from build123d import *

# Parameters (mm, degrees)
ESQUISSE3_R          = 17.5
EXTRUSION1_DEPTH     = 10
EXTRUSION3_START     = -35
EXTRUSION3_OUTLINE_R = 10
EXTRUSION3_DEPTH     = 7
ESQUISSE7_W          = 50
ESQUISSE7_H          = 50
EXTRUSION4_DEPTH     = 7
CONG_1_R             = 10


# Read off the part's stored shape, not the designer's step: Extrusion3
with BuildPart() as part:
    # Esquisse1 → Révol.-Mince1 (revolve)
    with BuildSketch(Plane.XY):
        with BuildLine():
            ThreePointArc((0, -30), (30, 0), (0, 30))
            Line((0, 30), (0, 31))
            ThreePointArc((0, 31), (31, 0), (0, -31))
            Line((0, -31), (0, -30))
        make_face()
    revolve(axis=Axis((0, 52.542035398, 0), (0, -1, 0)))

    # Esquisse3 → Extrusion1 (add)
    with BuildSketch(Plane.XY.offset(20)):
        with Locations(Location((0, 0, 0), (0, 0, 180))):
            Circle(ESQUISSE3_R)
    extrude(amount=EXTRUSION1_DEPTH)

    # Extrusion3 outline → Extrusion3 (add)
    with BuildSketch(Plane(origin=(0, 0, 0), x_dir=(1, 0, 0), z_dir=(0, 1, 0)).offset(EXTRUSION3_START)):
        Circle(EXTRUSION3_OUTLINE_R)
    extrude(amount=EXTRUSION3_DEPTH)

    # Esquisse7 → Extrusion4 (add)
    with BuildSketch(Plane.XZ.offset(35)):
        Rectangle(ESQUISSE7_W, ESQUISSE7_H)
    extrude(amount=EXTRUSION4_DEPTH)

    # Congé1
    cong_1_edges = [part.edges().sort_by_distance(p)[0] for p in [
        (25, -38.5, -25),
        (25, -38.5, 25),
        (-25, -38.5, 25),
        (-25, -38.5, -25),
    ]]
    fillet(cong_1_edges, radius=CONG_1_R)


solid = part.part
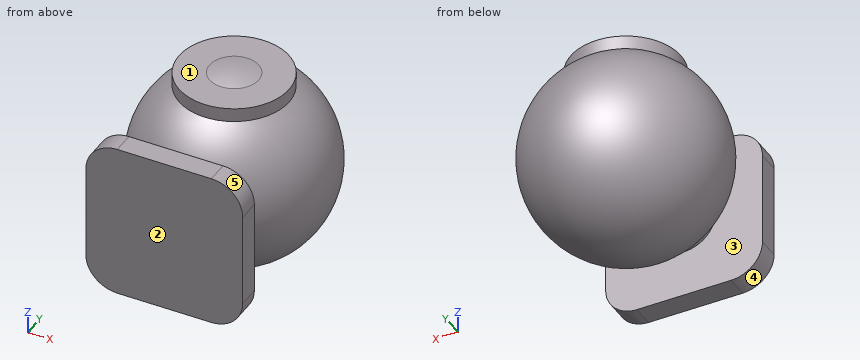
The listing builds one solid part. Answer for the finished solid, in the listing's coordinates (mm). Face numbers are marked on the shaded views. A direction names the side the tool comes from. Coordinates: 2 decimals unless noted, no trailing zeros. Loops run counter-clockwise (first coordinate to the right, second up) from the corner with the lowest first, then second, coordinate; pieces in that order, holes last. Notation, with made-up numbers: M 10.5,-29.75 L 42.5,-29.75 A16 ccw 42.5,-22.75 Z; hole C -20.5,9.5 d5. An arc over 180 degrees is marked long. Answer in a Markdown table with one row per item.
1) Find section A-A (z = 0). Determine the outline of the cut face in (x, y), then the cut area to 3 significant figures.
Answers below:
| item | result |
|---|---|
| outline | M -25,-42 L 25,-42 L 25,-35 L 10,-35 L 10,-29.34 A31 ccw long -10,-29.34 L -10,-35 L -25,-35 Z; hole M -10,-28.28 L -10,-28 L 10,-28 L 10,-28.28 A30 ccw long Z |
| area | 661 mm^2 |
2) Given pin 1 (5.5 mm diameter, centred on y = -38.5, z = 0, fed in from -X); pin 2 (17.5 mm diameter, centred on x = 8, y = 1.5, fed in from -Z); pin 3 (12 mm diameter, centred on x = -16, z = -13.5, fed in from +Y), each flat-ended and moving along its own axis, determine where each tip first touches the part or whether it passes through.
Answers below:
| item | result |
|---|---|
| pin 1 | x = -25 |
| pin 2 | z = -31 |
| pin 3 | y = 27.17 |
3) Which of the six approach directions +Z, -Z, +X, -X, +Y, -Y give full straight-line access (tool end or side, diameter ignored) to the marked faces 4 and 5?
Answers below:
| item | result |
|---|---|
| face 4 | -Z, -X, -Y |
| face 5 | +Z, +X, -Y |
4) Find the intervals of material crossed by probe 1 along Y at (x, z) = (-4, -12); probe 2 along Y at (x, z) = (-13, -16.5); probe 3 along Z at (x, y) = (-4, 5.5), in increasing order.
Answers below:
| item | result |
|---|---|
| probe 1 | -42 to -35, -28.3 to -27.2, 27.2 to 28.3 |
| probe 2 | -42 to -35, -22.8 to -21.42, 21.42 to 22.8 |
| probe 3 | -30.24 to -29.22, 20 to 30.24 |
5) Find section B-B (x = 23.5). Determine the outline of the cut face in (y, z).
Answers below:
| item | result |
|---|---|
| outline | M -42,-20.27 L -35,-20.27 L -35,20.27 L -42,20.27 Z; C 0,0 d40.44; hole C 0,0 d37.3 |
6) Determine the mould class of the marked faces 1, 2 and 3 for opening direction Y: released by +Y, released by -Y, zero draft, split by the parting line, or undercut.
Answers below:
| item | result |
|---|---|
| face 1 | zero draft |
| face 2 | released by -Y |
| face 3 | undercut |
7) Find section C-C (y = 0). Determine the outline of the cut face in (x, z), then the cut area to 3 significant figures.
Answers below:
| item | result |
|---|---|
| outline | M -17.5,25.59 A31 ccw long 17.5,25.59 L 17.5,30 L 7.81,30 A31 ccw -7.81,30 L -17.5,30 Z; hole M -17.5,20 L -17.5,24.37 A30 ccw long 17.5,24.37 L 17.5,20 Z |
| area | 515 mm^2 |
8) Find section D-D (x = 0). Determine the outline of the cut face in (y, z), then the cut area to 3 significant figures.
Answers below:
| item | result |
|---|---|
| outline | M -42,-25 L -35,-25 L -35,-10 L -29.34,-10 A31 ccw long 17.5,25.59 L 17.5,30 L 7.81,30 A31 ccw -7.81,30 L -17.5,30 L -17.5,25.59 A31 ccw -29.34,10 L -35,10 L -35,25 L -42,25 Z; hole M -28.28,-10 A30 ccw long 17.5,24.37 L 17.5,20 L -17.5,20 L -17.5,24.37 A30 ccw -28.28,10 L -28,10 L -28,-10 Z |
| area | 984 mm^2 |
